from build123d import *

# Parameters (mm, degrees)
F0_R     = 190.5
F1_DEPTH = 88.9
F2_R     = 76.2
F3_DEPTH = 25.4
F4_R     = 76.2
F5_DEPTH = 25.4
F6_R     = 7.9375
F7_DEPTH = 127
F8_R     = 44.45


with BuildPart() as f1:
    # F0 (on Front) → F1 (new body, symmetric)
    with BuildSketch(Plane.XZ):
        Circle(F0_R)
    extrude(amount=F1_DEPTH, both=True)

    # F2 (on face) → F3 (cut)
    with BuildSketch(Plane.XZ.offset(88.9)):
        Circle(F2_R)
    extrude(amount=-F3_DEPTH, mode=Mode.SUBTRACT)

    # F4 (on face) → F5 (cut)
    with BuildSketch(Plane(origin=(0, 88.9, 0), x_dir=(-1, 0, 0), z_dir=(0, 1, 0))):
        Circle(F4_R)
    extrude(amount=-F5_DEPTH, mode=Mode.SUBTRACT)

    # F6 (on face) → F7 (cut, symmetric)
    with BuildSketch(Plane.XZ.offset(63.5)):
        Circle(F6_R)
    extrude(amount=F7_DEPTH, both=True, mode=Mode.SUBTRACT)

    # F8
    f8_edges = [f1.edges().sort_by_distance(p)[0] for p in [
        (-190.5, 88.9, 0),
        (-190.5, -88.9, 0),
    ]]
    fillet(f8_edges, radius=F8_R)


solid = f1.part
CAD build for the part. Positions are in the model's coordinates, mm. A direction names the side the tool comes from. Round coordinates to 2 decimals unless told otherwise and drop trailing zeros. Write each loop counter-clockwise with the first axis right and the second up, starting at its lowest first coordinate (ties: lowest second). Pieces come first, ordered by that corner, then holes.
(1) Drop flat-ended pins along their axis: P1, Ø6, axis at x = 23, y = 5.5, coming from the -Z side; P2, Ø5, axis at x = -135, y = 22, coming from the +Z side; P3, Ø1.5, axis at x = -27, y = -70.5, coming from the +Z side. Give the stop position or say it passes through.
(2) Slice it at A-A, the plane z = 0. Write the cut outline in (x, y).
(3) Slice it at C-C, the plane y = 12. Write the cut outline in (x, z) (1 decimal).
(4) Probe line 1 along Z through (x, y) = (0, 12); line 2 along Y through (x, z) = (-24, -66); line 3 along Z through (x, y) = (0, 74). List the from-to ranges inside material, lowest first.
(5) Slice it at D-D, the plane y = 55. Write the cut outline in (x, z) (1 decimal), and give its area (3 significant figures).
(6) 3-axis set-ups, long thin cutter, end or side, ignore diameter. For faces 5 (the face through (63, -88.9, -63)), 6 (the face through (60.47, 76.378, -46.367)): which of +Z, -Z, +X, -X, +Y, -Y reach the whole face in a straight line?
(7) Mould opens along X. For faces 1 (the face through (63, 88.9, -63)), 2 (the face through (-151.17, -0.62, -115.92)), 3 (the face through (-60.47, -76.378, -46.367)), 4 (the face through (16, -63.5, 1)) say: pulls with the +X half, pulls with the -X half, needs draft (parallel to the pull), parting line crosses it, or undercut.
(8) Slice it at B-B, the plane x = 0. Write the cut outline in (y, z), and give its area (3 significant figures).
From the geometry:
1. P1: stops at z = -189.45
1. P2: stops at z = 136.87
1. P3: stops at z = 180.6
2. outline: (-190.5, -44.45) arc R44.45 ccw to (-146.05, -88.9) - (-76.2, -88.9) - (-76.2, -63.5) - (-7.94, -63.5) - (-7.94, 63.5) - (-76.2, 63.5) - (-76.2, 88.9) - (-146.05, 88.9) arc R44.45 ccw to (-190.5, 44.45) - close; (7.94, -63.5) - (76.2, -63.5) - (76.2, -88.9) - (146.05, -88.9) arc R44.45 ccw to (190.5, -44.45) - (190.5, 44.45) arc R44.45 ccw to (146.05, 88.9) - (76.2, 88.9) - (76.2, 63.5) - (7.94, 63.5) - close
3. outline: circle Ø381 at (0, 0); hole circle Ø15.9 at (0, 0)
4. line 1: z = -190.5 to -7.94, 7.94 to 190.5
4. line 2: y = -63.5 to 63.5
4. line 3: z = -179.26 to -76.2, 76.2 to 179.26
5. outline: circle Ø378.5 at (0, 0); hole circle Ø15.9 at (0, 0)
5. area: 112,000 mm2
6. face 5: +Z, -Z, +X, -X, -Y
6. face 6: +Y
7. face 1: needs draft
7. face 2: parting line crosses it
7. face 3: undercut
7. face 4: undercut
8. outline: (-88.9, -146.05) arc R44.45 ccw to (-44.45, -190.5) - (44.45, -190.5) arc R44.45 ccw to (88.9, -146.05) - (88.9, -76.2) - (63.5, -76.2) - (63.5, -7.94) - (-63.5, -7.94) - (-63.5, -76.2) - (-88.9, -76.2) - close; (-88.9, 76.2) - (-63.5, 76.2) - (-63.5, 7.94) - (63.5, 7.94) - (63.5, 76.2) - (88.9, 76.2) - (88.9, 146.05) arc R44.45 ccw to (44.45, 190.5) - (-44.45, 190.5) arc R44.45 ccw to (-88.9, 146.05) - close
8. area: 56,300 mm2
